Source: CAD feature listing. Evaluate the final solid. Frame: model axes, mm. A direction names the side the tool comes from. Round coordinates to 2 decimals unless told otherwise and drop trailing zeros. Loops run counter-clockwise (first coordinate to the right, second up) from the corner with the lowest first, then second, coordinate; pieces in that order, holes last.
Item 1: Section query A-A on z = 49. Return loops of the section in (x, y), then the cut area to 3 significant figures.
Item 2: Ray query, L1, parallel to Y at x = 34, z = 34; L2, parallel to Z at x = -73.5, y = -65; L3, parallel to Z at x = -30.5, y = 2.5. Return the intervals inside material, ascending.
Item 3: Section query C-C on x = 69. Give the number of separate pieces and of enclosed holes in the cut face, then the cut area to 3 significant figures.
Item 4: Pull-direction query (Y, two-part tool) for faces 1 (the cylindrical face through (-1.4, -65.3, 71)), 2 (the cylindrical face through (1.4, -1.985, 32.524)), 3 (the flat face through (1, -41, 16.05)); classes: released by +Y, released by -Y, zero draft, split by the parting line, or undercut.
Item 5: Section query B-B on z = 62.5. Return loops of the section in (x, y), then the cut area to 3 significant figures.
Item 6: Section query D-D on z = -2.5. Return loops of the section in (x, y), then the cut area to 3 significant figures.
Item 7: Access query for faces 4 (the flat face through (1.4, -56.506, 52.213)), 5 (the flat face through (1, 4, 31.283)), 6 (the flat face through (1, -2.75, 0)), 7 (the cylindrical face through (-1.4, -13.71, 71.38)). Directions: +Z, -Z, +X, -X, +Y, -Y. A direction counts if a zero-diameter tool reaches every point of the face in a straight line with its end or side. Return the directions, or none.
Item 8: First-contact query: P1, Ø1, axis at x = 0, y = -41, coming from the -Z side; P2, Ø3, axis at x = 15, y = 3.5, coming from the +Z side; P3, Ø3, axis at y = -13.8, z = 69.38, coming from the +X side; P4, Ø6, axis at x = -58.5, y = -60.5, coming from the +Z side. Flat tips, straight axial feed; report the tip coordinate or a pass-through.
```python
from build123d import *

# Parameters (mm, degrees)
SKETCH2_R           = 2
BOSS_EXTRUDE1_DEPTH = 100
FILLET1_R           = 5


with BuildPart() as part:
    # Sketch2 → Boss-Extrude1 (new body, symmetric)
    with BuildSketch(Plane(origin=(0, 0, 0), x_dir=(0, 0, -1), z_dir=(1, 0, 0))):
        with BuildLine():
            Line((11.05, 12.25), (-11.05, 12.25))
            Line((-11.05, 12.25), (-31.283333333, 12.25))
            Line((-31.283333333, 12.25), (-31.283333333, -2.985208333))
            Line((-31.283333333, -2.985208333), (-69.383333333, -8.788333333))
            ThreePointArc((-69.383333333, -8.788333333), (-73.686594127, -13.796666667), (-69.383333333, -18.805))
            Line((-69.383333333, -18.805), (-35.516666667, -23.963333333))
            add(Edge.make_bspline(
                [(-35.516666667, -23.963333333), (-27.05, -25.252916667), (-27.05, -52.67375), (-35.516666667, -53.963333333)],
                knots=[0, 0, 0, 0, 1, 1, 1, 1], degree=3))
            Line((-35.516666667, -53.963333333), (-69.383333333, -59.121666667))
            ThreePointArc((-69.383333333, -59.121666667), (-75.036285741, -65.700833333), (-69.383333333, -72.28))
            Line((-69.383333333, -72.28), (-31.283333333, -72.28))
            Line((-31.283333333, -72.28), (-16.05, -72.28))
            Line((-16.05, -72.28), (-16.05, -13.796666667))
            add(Edge.make_bspline(
                [(-11.05, -2.75), (-16.05, -2.75), (-16.05, -13.796666667)],
                knots=[0, 0, 0, 1, 1, 1], degree=2))
            Line((-11.05, -2.75), (11.05, -2.75))
            Line((11.05, -2.75), (11.05, 12.25))
        make_face()
        with Locations((-35.516666667, -13.796666667)):
            Circle(SKETCH2_R, mode=Mode.SUBTRACT)
        with Locations((-69.383333333, -13.796666667)):
            Circle(SKETCH2_R, mode=Mode.SUBTRACT)
        with Locations((-35.516666667, -64.121666667)):
            Circle(SKETCH2_R, mode=Mode.SUBTRACT)
        with Locations((-69.383333333, -64.121666667)):
            Circle(SKETCH2_R, mode=Mode.SUBTRACT)
    extrude(amount=BOSS_EXTRUDE1_DEPTH, both=True)

    # Fillet1
    fillet1_edges = [part.edges().sort_by_distance(p)[0] for p in [
        (0, -72.28, 16.05),
        (0, -2.985208333, 31.283333333),
        (0, 12.25, 31.283333333),
        (0, 12.25, -11.05),
    ]]
    fillet(fillet1_edges, radius=FILLET1_R)


solid = part.part
```
Data:
1. outline: (-100, -72.28) - (100, -72.28) - (100, -56.02) - (-100, -56.02) - close; (-100, -21.91) - (100, -21.91) - (100, -5.68) - (-100, -5.68) - close
1. area: 6,500 mm2
2. L1: y = -72.28 to -65.43, -62.82 to -53.41, -24.52 to -15.1, -12.49 to -3.14
2. L2: z = 16.05 to 33.72, 37.31 to 67.59, 71.18 to 75
2. L3: z = -11.05 to 31.28
3. separate pieces: 1
3. enclosed holes: 4
3. area: 2,920 mm2
4. face 1: undercut
4. face 2: released by +Y
4. face 3: zero draft
5. outline: (-100, -72.28) - (100, -72.28) - (100, -58.07) - (-100, -58.07) - close; (-100, -19.85) - (100, -19.85) - (100, -7.74) - (-100, -7.74) - close
5. area: 5,260 mm2
6. outline: (-100, -2.75) - (100, -2.75) - (100, 12.25) - (-100, 12.25) - close
6. area: 3,000 mm2
7. face 4: +Z, +X, -X
7. face 5: +Z, +X, -X, +Y
7. face 6: -Z, +X, -X, -Y
7. face 7: +X, -X
8. P1: stops at z = 16.05
8. P2: stops at z = 31.28
8. P3: passes through
8. P4: stops at z = 74.66
